```python
from build123d import *

# Parameters (mm, degrees)
ESBO_O1_W                = 150
ESBO_O1_H                = 150
RESSALTO_EXTRUS_O1_DEPTH = 5
ESBO_O2_R                = 5
RESSALTO_EXTRUS_O2_DEPTH = 15
ESBO_O4_R                = 1.5
CORTE_EXTRUS_O1_DEPTH    = 15


with BuildPart() as part:
    # Esboço1 → Ressalto-extrusão1 (new body)
    with BuildSketch(Plane(origin=(0, 0, 0), x_dir=(1, 0, 0), z_dir=(0, 1, 0))):
        with Locations((-258.939300439, 168.363905829)):
            Rectangle(ESBO_O1_W, ESBO_O1_H)
    extrude(amount=RESSALTO_EXTRUS_O1_DEPTH)

    # Esboço2 → Ressalto-extrusão2 (add)
    with BuildSketch(Plane(origin=(0, 0, 0), x_dir=(-1, 0, 0), z_dir=(0, -1, 0))):
        with Locations(Location((291.439300439, 135.863905829, 0), (0, 0, 270))):
            Circle(ESBO_O2_R)
        with Locations(Location((226.439300439, 135.863905829, 0), (0, 0, 270))):
            Circle(ESBO_O2_R)
        with Locations(Location((291.439300439, 200.863905829, 0), (0, 0, 270))):
            Circle(ESBO_O2_R)
        with Locations(Location((226.439300439, 200.863905829, 0), (0, 0, 270))):
            Circle(ESBO_O2_R)
    extrude(amount=RESSALTO_EXTRUS_O2_DEPTH)

    # Esboço4 → Corte-extrusão1 (cut)
    with BuildSketch(Plane(origin=(0, -15, 0), x_dir=(-1, 0, 0), z_dir=(0, -1, 0))):
        with Locations(Location((291.439300439, 135.863905829, 0), (0, 0, 90))):
            Circle(ESBO_O4_R)
        with Locations(Location((226.439300439, 135.863905829, 0), (0, 0, 90))):
            Circle(ESBO_O4_R)
        with Locations(Location((291.439300439, 200.863905829, 0), (0, 0, 90))):
            Circle(ESBO_O4_R)
        with Locations(Location((226.439300439, 200.863905829, 0), (0, 0, 90))):
            Circle(ESBO_O4_R)
    extrude(amount=-CORTE_EXTRUS_O1_DEPTH, mode=Mode.SUBTRACT)


solid = part.part
```
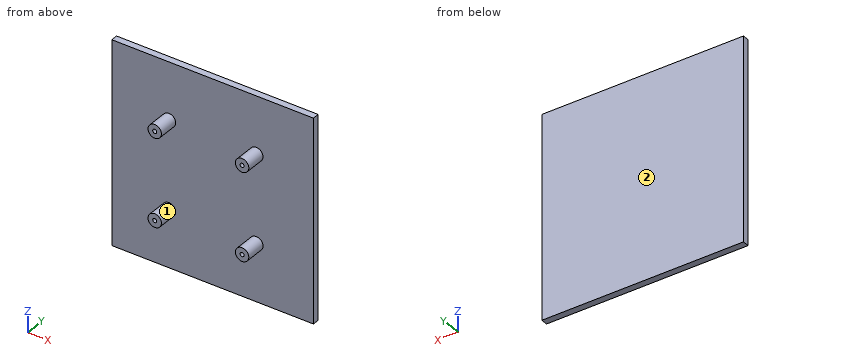
Source: CAD feature listing. Evaluate the final solid. Frame: model axes, mm. Face numbers are marked on the shaded views. Coordinates: 2 decimals unless noted, no trailing zeros. Write each loop counter-clockwise with the first axis right and the second up, starting at its lowest first coordinate (ties: lowest second). Pieces come first, ordered by that corner, then holes. Notation, with made-up numbers: (12.25, 37) -> (18.25, 37) arc R22 ccw to (18.25, 50) -> close; hole circle Ø5 at (11, -18). An arc over 180 degrees is marked (long way). Return JSON: item names as keys, results as strings. Group by question number.
1) Contact query for flat-ended pins moving along their axis: P1, Ø10, axis at x = -314, y = -6.5, coming from the -Z side; P2, Ø2.5, axis at x = -292, z = -135.5, coming from the -Y side; P3, Ø5, axis at x = -213.5, z = -182.5, coming from the -Y side. Output: stop coordinate, or through.
2) Section query B-B, the plane x = -280. Return loops of the section in (y, z), plus the area to 3 significant figures.
3) Section query A-A, the plane y = -3.25. Return loops of the section in (x, z), plus the area to 3 significant figures.
4) Ray query, line 1 along X through (y, z) = (-2.5, -134.5) (3 decimals); line 2 along Y through (x, z) = (-301.5, -159.5); line 3 along Z through (x, y) = (-294, -10.5). Return the intervals inside material, ascending.
5) Mould query, pull axis X, two halves, no side actions, for the marked faces 1 and 2. Classes: +X half, -X half, draft (parallel to the pull), parting line (faces both ways), or undercut.
6) Section query C-C, the plane z = -186.5. Return loops of the section in (x, y), plus the area to 3 significant figures.
From the geometry:
{
 "1": {"P1": "through", "P2": "y = -15", "P3": "y = 0"},
 "2": {"outline": "(0, -243.36) -> (5, -243.36) -> (5, -93.36) -> (0, -93.36) -> close", "area": "750 mm²"},
 "3": {"outline": "circle Ø10 at (-291.44, -200.86); circle Ø10 at (-291.44, -135.86); circle Ø10 at (-226.44, -200.86); circle Ø10 at (-226.44, -135.86); hole circle Ø3 at (-291.44, -200.86); hole circle Ø3 at (-291.44, -135.86); hole circle Ø3 at (-226.44, -200.86); hole circle Ø3 at (-226.44, -135.86)", "area": "286 mm²"},
 "4": {"line 1": "-296.25 to -292.064, -290.815 to -286.629, -231.25 to -227.064, -225.815 to -221.629", "line 2": "0 to 5", "line 3": "-205.16 to -196.57, -140.16 to -131.57"},
 "5": {"face 1": "undercut", "face 2": "draft"},
 "6": {"outline": "(-333.94, 0) -> (-183.94, 0) -> (-183.94, 5) -> (-333.94, 5) -> close", "area": "750 mm²"}
}
